CAD build for the part. Positions are in the model's coordinates, mm. Round coordinates to 2 decimals unless told otherwise and drop trailing zeros. Write each loop counter-clockwise with the first axis right and the second up, starting at its lowest first coordinate (ties: lowest second). Pieces come first, ordered by that corner, then holes. Notation, with made-up numbers: (86, 41) - (92, 41) arc R23 ccw to (92, 57) - close; hole circle Ø4 at (-27.75, 30). An arc over 180 degrees is marked (long way). Answer in a Markdown table with one row per item.
```python
from build123d import *

# Parameters (mm, degrees)
ESQUISSE1_R        = 10
ESQUISSE1_W        = 40
ESQUISSE1_H        = 40
BOSS_EXTRU_1_DEPTH = 10
CONG_1_R           = 10
CONG_2_R           = 20


with BuildPart() as part:
    # Esquisse1 → Boss.-Extru.1 (new body)
    with BuildSketch(Plane(origin=(0, 0, 0), x_dir=(0, 0, -1), z_dir=(1, 0, 0))):
        with BuildLine():
            Line((0, 30), (-764.641016151, 30))
            Line((-764.641016151, 30), (-1181.961524227, -692.820323028))
            Line((-1181.961524227, -692.820323028), (-1173.301270189, -697.820323028))
            Line((-1173.301270189, -697.820323028), (-1153.301270189, -663.179306876))
            Line((-1153.301270189, -663.179306876), (-1118.660254038, -683.179306876))
            Line((-1118.660254038, -683.179306876), (-1138.660254038, -717.820323028))
            Line((-1138.660254038, -717.820323028), (-1130, -722.820323028))
            Line((-1130, -722.820323028), (-730, -30))
            Line((-730, -30), (0, -30))
            ThreePointArc((0, -30), (30, 0), (0, 30))
        make_face()
        Circle(ESQUISSE1_R, mode=Mode.SUBTRACT)
        with Locations((-60, 0)):
            Rectangle(ESQUISSE1_W, ESQUISSE1_H, mode=Mode.SUBTRACT)
        Polygon((-737.113248654, 22.320508076), (-771.754264805, 2.320508076), (-751.754264805, -32.320508076), (-717.113248654, -12.320508076), align=None, mode=Mode.SUBTRACT)
    extrude(amount=BOSS_EXTRU_1_DEPTH)

    # Congé1
    cong_1_edges = [part.edges().sort_by_distance(p)[0] for p in [
        (5, -692.820323028, 1181.961524227),
        (5, -722.820323028, 1130),
    ]]
    fillet(cong_1_edges, radius=CONG_1_R - 0.0001)  # a hair under: the kernel refuses the full size

    # Congé2
    cong_2_edges = [part.edges().sort_by_distance(p)[0] for p in [
        (5, -30, 730),
        (5, 30, 764.641016151),
    ]]
    fillet(cong_2_edges, radius=CONG_2_R)


solid = part.part
```
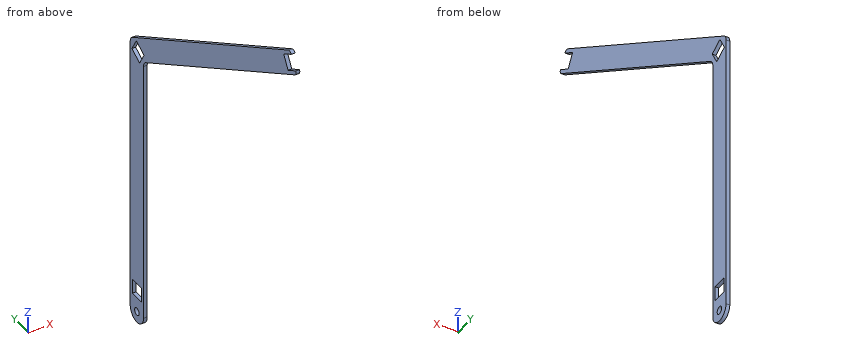
Q1. Flat gauge pins, fed straight in: pin 1 (2 mm diameter, centred on x = 2.5, y = -401, fed in from +Z); pin 2 (3 mm diameter, centred on x = 2, y = -122.5, fed in from +Z); pin 3 (1.5 mm diameter, centred on x = 2, z = 868.5, fed in from +Y). Where does each tip first touch, or does it go through?
Computed:
| item | result |
|---|---|
| pin 1 | stops at z = 1014.06 |
| pin 2 | stops at z = 853.55 |
| pin 3 | stops at y = -148.59 |
Q2. Saw through at B-B on z = 152. List the corners of the cut face in (x, y).
Computed:
| item | result |
|---|---|
| outline | (0, -30) - (10, -30) - (10, 30) - (0, 30) - close |
Q3. Saw through at C-C on y = -646.5. List the corners of the cut face in (x, z).
Computed:
| item | result |
|---|---|
| outline | (0, 1085.94) - (10, 1085.94) - (10, 1155.22) - (0, 1155.22) - close |
Q4. Saw through at A-A on x = 8.5. Count the separate pieces of the cut face and the enclosed holes in it, then the cut area to 3 significant figures.
Computed:
| item | result |
|---|---|
| separate pieces | 1 |
| enclosed holes | 3 |
| area | 90,100 mm2 |
Q5. Drill centre lines: line 1 (Y direction, x = 8, z = 0); line 2 (Z direction, x = 4.25, y = -3); line 3 (Y direction, x = 9.75, z = 659). Where is each one in solid material? Low to high.
Computed:
| item | result |
|---|---|
| line 1 | y = -30 to -10, 10 to 30 |
| line 2 | z = -29.85 to -9.54, 9.54 to 40, 80 to 722.49, 768.68 to 783.69 |
| line 3 | y = -30 to 30 |
